Read the model definition and answer for the solid it produces. Units are mm, in the model's axes. Give positions to 0.01 mm unless a question says otherwise; leave off trailing zeros. Order: outer loops, then holes, each group sorted by start corner. A loop starts at its lowest first (then second) coordinate and runs counter-clockwise, first axis right, second up. Notation, with made-up numbers: (85, 3.25) -> (122, 3.25) arc R15 cw to (122, 21.25) -> close; hole circle Ø5 at (49, 68.5). An arc over 180 degrees is marked (long way). One line per item, written item: value. Start each with the question number.
Autodesk Inventor part; units mm, degrees
ref_plane "YZ Plane" through (0, 0, 0) normal (1, 0, 0) x (0, 1, 0)
ref_plane "XZ Plane" through (0, 0, 0) normal (0, 1, 0) x (-1, 0, 0)
ref_plane "XY Plane" through (0, 0, 0) normal (0, 0, 1) x (1, 0, 0)
sketch "Sketch1" plane through (2835.9464, 0.127, -1682.1632) normal (0, 1, 0) x (1, 0, 0)
  line L0 (0, -1676.4) -> (50.8001, -1676.4)
  line L1 (50.8001, -1676.4) -> (50.8001, -50.8)
  line L2 (50.8001, -50.8) -> (758.8544, -50.8)
  line L3 (758.8544, -50.8) -> (758.7571, 0) construction
  line L4 (758.7571, 0) -> (0, 0)
  line L5 (0, 0) -> (0, -1676.4)
  line L6 (758.8544, -50.8) -> (758.8544, 0)
  line L7 (758.8544, -50.8) -> (809.6544, -50.8) construction
  line L8 (758.8544, 0) -> (0, 0)
  line L9 (0, 0) -> (0, -1676.4)
  line L10 (0, -1676.4) -> (50.8001, -1676.4)
  line L11 (50.8001, -1676.4) -> (50.8001, -50.8)
  line L12 (50.8001, -50.8) -> (758.8544, -50.8)
  point P0 (-2835.9464, -1682.1632)
  dimension "d0" = 90
  dimension "d1" = 90
  dimension "d2" = 90
extrude "Extrusion1" add sketch "Sketch1" against normal blind 0.127
properties part number "protected zone tape Red"
Item 1: Find section B-B on x = 3422. Write down the section's boundary in (y, z).
Item 2: Find the intervals of material crossed by line 1 (Z direction, x = 3495.5, y = 0.05), in increasing order. Write a range as from..to.
Item 3: Find section C-C on z = -498.5. Write down the section's boundary in (x, y).
Item 4: Find section A-A on y = 0.05. Write down the section's boundary in (x, z), then the cut area to 3 significant figures.
Checks:
1. outline: (0, -1682.16) -> (0.13, -1682.16) -> (0.13, -1631.36) -> (0, -1631.36) -> close
2. line 1: -1682.16..-1631.36
3. outline: (2835.95, 0) -> (2886.75, 0) -> (2886.75, 0.13) -> (2835.95, 0.13) -> close
4. outline: (2835.95, -1682.16) -> (3594.8, -1682.16) -> (3594.8, -1631.36) -> (2886.75, -1631.36) -> (2886.75, -5.76) -> (2835.95, -5.76) -> close
4. area: 121,000 mm2
